Work out the finished part from the listing and answer in its coordinate system (mm). A direction names the side the tool comes from. Round coordinates to 2 decimals unless told otherwise and drop trailing zeros. Loops run counter-clockwise (first coordinate to the right, second up) from the corner with the lowest first, then second, coordinate; pieces in that order, holes last.
```python
from build123d import *

# Parameters (mm, degrees)
BOSS_EXTRUDE1_DEPTH = 5
BOSS_EXTRUDE2_DEPTH = 5


with BuildPart() as part:
    # Sketch1 → Boss-Extrude1 (new body)
    with BuildSketch(Plane.XY):
        Polygon((14.3, 12.85), (14.3, 11.95), (20.4, 11.95), (20.4, -11.75), (-20.4, -11.75), (-20.4, 11.95), (-14.3, 11.95), (-14.3, 12.85), (-21.3, 12.85), (-21.3, -12.85), (21.3, -12.85), (21.3, 12.85), align=None)
    extrude(amount=BOSS_EXTRUDE1_DEPTH)

    # Sketch1_3 → Boss-Extrude2 (add)
    with BuildSketch(Plane.XY):
        with BuildLine():
            Line((14.190689839, -14.299541794), (13.190689839, -14.299541794))
            Line((13.190689839, -14.299541794), (13.190689839, -15.85))
            ThreePointArc((13.190689839, -15.85), (16.690689839, -19.35), (20.190689839, -15.85))
            Line((20.190689839, -15.85), (20.190689839, -12.85))
            Line((20.190689839, -12.85), (19.190689839, -12.85))
            Line((19.190689839, -12.85), (19.190689839, -15.85))
            ThreePointArc((19.190689839, -15.85), (16.690689839, -18.35), (14.190689839, -15.85))
            Line((14.190689839, -15.85), (14.190689839, -14.299541794))
        make_face()
    extrude(amount=BOSS_EXTRUDE2_DEPTH)


solid = part.part
```
1. Find section D-D (x = -8). Write down the section's boundary in (y, z).
Answer key:
outline: (-12.85, 0) - (-11.75, 0) - (-11.75, 5) - (-12.85, 5) - close
2. Determine the mould class of faces 5 (the face through (21, -12.85, 2)), 6 (the face through (-21.3, 0, 2)), 7 (the face through (0, -11.75, 2)) for opening direction X: +X half, -X half, draft (parallel to the pull), parting line (faces both ways), or undercut.
Answer key:
face 5: draft
face 6: -X half
face 7: undercut
3. Find section C-C (x = 15). Write down the section's boundary in (y, z), then the cut area to 3 significant figures.
Answer key:
outline: (-18.91, 0) - (-17.69, 0) - (-17.69, 5) - (-18.91, 5) - close; (-12.85, 0) - (-11.75, 0) - (-11.75, 5) - (-12.85, 5) - close; (11.95, 0) - (12.85, 0) - (12.85, 5) - (11.95, 5) - close
area: 16.1 mm2
4. Find section A-A (y = -3). Write down the section's boundary in (x, z), then the cut area to 3 significant figures.
Answer key:
outline: (-21.3, 0) - (-20.4, 0) - (-20.4, 5) - (-21.3, 5) - close; (20.4, 0) - (21.3, 0) - (21.3, 5) - (20.4, 5) - close
area: 9.00 mm2
5. Which of the six approach directions +Z, -Z, +X, -X, +Y, -Y give full straight-line access (tool end or side, diameter ignored) to faces 1 (the face through (19.191, -14, 2)), 2 (the face through (1.5, -12.7, 0)), 3 (the face through (20.191, -14, 2)), 4 (the face through (14, -14.3, 2))?
Answer key:
face 1: +Z, -Z
face 2: -Z, +X, -X, +Y, -Y
face 3: +Z, -Z, +X, -Y
face 4: +Z, -Z, -X
6. Consider probe 1 along X at (y, z) = (-11, 4.6); probe 2 along Y at (x, z) = (18.5, 1.45); probe 3 along X at (y, z) = (-13.5, 4.5). Determine where each line is inside the solid, lowest interval first.
Answer key:
probe 1: x = -21.3 to -20.4, 20.4 to 21.3
probe 2: y = -18.85 to -17.58, -12.85 to -11.75, 11.95 to 12.85
probe 3: x = 19.19 to 20.19
7. Find section B-B (z = 1.7). Write down the section's boundary in (x, y).
Answer key:
outline: (-21.3, -12.85) - (19.19, -12.85) - (19.19, -15.85) arc R2.5 cw to (14.19, -15.85) - (14.19, -14.3) - (13.19, -14.3) - (13.19, -15.85) arc R3.5 ccw to (20.19, -15.85) - (20.19, -12.85) - (21.3, -12.85) - (21.3, 12.85) - (14.3, 12.85) - (14.3, 11.95) - (20.4, 11.95) - (20.4, -11.75) - (-20.4, -11.75) - (-20.4, 11.95) - (-14.3, 11.95) - (-14.3, 12.85) - (-21.3, 12.85) - close
8. Given pin 1 (1 mm diameter, centred on x = 5, z = 1.5, fed in from +Y); pin 2 (0.8 mm diameter, centred on y = -15, z = 2, fed in from -X); pin 3 (1.2 mm diameter, centred on x = 20.5, z = 3.5, fed in from -Y); pin 4 (12 mm diameter, centred on x = -15.5, y = -1.5, fed in from -Z), each flat-ended and moving along its own axis, determine where each tip first touches the part or whether it passes through.
Answer key:
pin 1: stops at y = -11.75
pin 2: stops at x = 13.19
pin 3: stops at y = -17.25
pin 4: stops at z = 0
